Design review of the part built by this model. Coordinates are the model's own, in mm. Face numbers are marked on the shaded views. A direction names the side the tool comes from. Give positions to 0.01 mm unless a question says otherwise; leave off trailing zeros. Write each loop counter-clockwise with the first axis right and the second up, starting at its lowest first coordinate (ties: lowest second). Pieces come first, ordered by that corner, then holes. Notation, with made-up numbers: M -20,87 L -15,87 A25 ccw -15,120 Z; hole C 51.25,0 d1. An arc over 180 degrees is marked long. Answer in a Markdown table with one row per item.
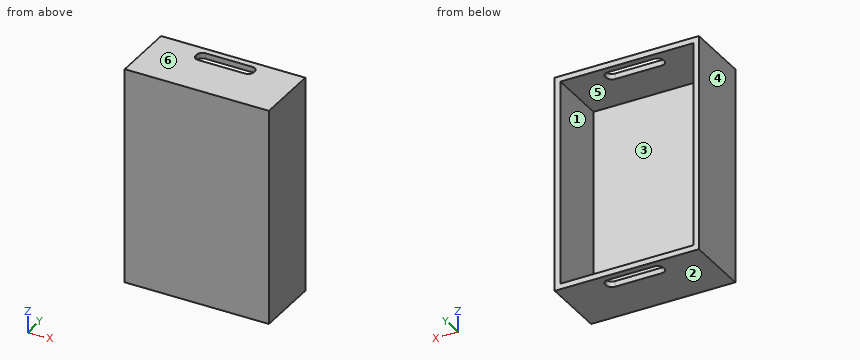
```python
from build123d import *

# Parameters (mm, degrees)
SKETCH1_W               = 385
SKETCH1_H               = 578
BOSS_EXTRUDE1_DEPTH     = 15
SKETCH2_W               = 15
SKETCH2_H               = 578
BOSS_EXTRUDE2_DEPTH     = 157.5
SKETCH3_W               = 355
SKETCH3_H               = 15
BOSS_EXTRUDE3_DEPTH     = 157.5
CUT_EXTRUDE1_DEPTH      = 634.16388084
CUT_EXTRUDE1_DEPTH_BACK = 634.16388084


with BuildPart() as part:
    # Sketch1 → Boss-Extrude1 (new body)
    with BuildSketch(Plane(origin=(0, 0, 0), x_dir=(1, 0, 0), z_dir=(0, 1, 0))):
        Rectangle(SKETCH1_W, SKETCH1_H)
    extrude(amount=BOSS_EXTRUDE1_DEPTH)

    # Sketch2 → Boss-Extrude2 (add)
    with BuildSketch(Plane(origin=(0, 15, 0), x_dir=(1, 0, 0), z_dir=(0, 1, 0))):
        with Locations((185, 0)):
            Rectangle(SKETCH2_W, SKETCH2_H)
    boss_extrude2 = extrude(amount=BOSS_EXTRUDE2_DEPTH)

    # Mirror1: Boss-Extrude2 across plane
    add(boss_extrude2.mirror(Plane(origin=(0, 0, 0), x_dir=(0, 0, 1), z_dir=(1, 0, 0))))

    # Sketch3 → Boss-Extrude3 (add)
    with BuildSketch(Plane(origin=(0, 15, 0), x_dir=(1, 0, 0), z_dir=(0, 1, 0))):
        with Locations((0, -281.5)):
            Rectangle(SKETCH3_W, SKETCH3_H)
    boss_extrude3 = extrude(amount=BOSS_EXTRUDE3_DEPTH)

    # Mirror2: Boss-Extrude3 across plane
    add(boss_extrude3.mirror(Plane.XY))

    # Sketch4 → Cut-Extrude1 (cut, two sides: drawn at the far end of the back side and taken through both)
    with BuildSketch(Plane.XY.offset(289).offset(-CUT_EXTRUDE1_DEPTH_BACK)):
        with BuildLine():
            Line((-64.034446869, 155), (60.965553131, 155))
            ThreePointArc((60.965553131, 155), (71.572154849, 150.606601718), (75.965553131, 140))
            Line((75.965553131, 140), (75.965553131, 135))
            ThreePointArc((75.965553131, 135), (71.572154849, 124.393398282), (60.965553131, 120))
            Line((60.965553131, 120), (-64.034446869, 120))
            ThreePointArc((-64.034446869, 120), (-74.641048586, 124.393398282), (-79.034446869, 135))
            Line((-79.034446869, 135), (-79.034446869, 140))
            ThreePointArc((-79.034446869, 140), (-74.641048586, 150.606601718), (-64.034446869, 155))
        make_face()
    extrude(amount=CUT_EXTRUDE1_DEPTH + CUT_EXTRUDE1_DEPTH_BACK, mode=Mode.SUBTRACT)


solid = part.part
```
1) To check wall thickness, follow probe 1 along X at (y, z) = (77.5, -117.5); probe 2 along Z at (x, y) = (-27, 16); probe 3 along Y at (x, z) = (116, 65.5). State the ranges of each line that lie inside material, in increasing order. Write a range as [from, to].
Geometry says:
| item | result |
|---|---|
| probe 1 | [-192.5, -177.5], [177.5, 192.5] |
| probe 2 | [-289, -274], [274, 289] |
| probe 3 | [0, 15] |
2) Add section C-C (y = 112.5). Write out the cut boundary in (x, z), and give its area (3 significant figures).
Geometry says:
| item | result |
|---|---|
| outline | M -192.5,-289 L 192.5,-289 L 192.5,289 L -192.5,289 Z; hole M -177.5,-274 L 177.5,-274 L 177.5,274 L -177.5,274 Z |
| area | 28,000 mm^2 |
3) Add section B-B (z = 32). Write out the cut boundary in (x, y).
Geometry says:
| item | result |
|---|---|
| outline | M -192.5,0 L 192.5,0 L 192.5,172.5 L 177.5,172.5 L 177.5,15 L -177.5,15 L -177.5,172.5 L -192.5,172.5 Z |
4) The part is to be moulded in two halves that separate along X. For the marked faces 3, 4, 5 and 6, say which applies: released by +X, released by -X, zero draft, split by the parting line, or undercut.
Geometry says:
| item | result |
|---|---|
| face 3 | undercut |
| face 4 | released by -X |
| face 5 | undercut |
| face 6 | zero draft |
5) Add section D-D (y = 146). Write out the cut boundary in (x, z).
Geometry says:
| item | result |
|---|---|
| outline | M -192.5,-289 L -77.78,-289 L -77.78,-274 L -177.5,-274 L -177.5,274 L -77.78,274 L -77.78,289 L -192.5,289 Z; M 74.71,-289 L 192.5,-289 L 192.5,289 L 74.71,289 L 74.71,274 L 177.5,274 L 177.5,-274 L 74.71,-274 Z |
6) Insertion check: P1, Ø1, axis at x = -100, z = -114.5, coming from the +Y side. The pin has a flat end and moves straight along its axis. Give the tip position at first contact, or say it passes through.
Geometry says:
| item | result |
|---|---|
| P1 | y = 15 |
7) For the marked faces 1 and 2, list the 3-axis set-ups (+Z, -Z, +X, -X, +Y, -Y) from which the entire face can be reached by the end or side of a thin tool; tool diameter is ignored.
Geometry says:
| item | result |
|---|---|
| face 1 | +Y |
| face 2 | -Z, +X, -X, +Y, -Y |
8) Add section A-A (x = 36). Write out the cut boundary in (y, z), and give its area (3 significant figures).
Geometry says:
| item | result |
|---|---|
| outline | M 0,-289 L 120,-289 L 120,-274 L 15,-274 L 15,274 L 120,274 L 120,289 L 0,289 Z; M 155,-289 L 172.5,-289 L 172.5,-274 L 155,-274 Z; M 155,274 L 172.5,274 L 172.5,289 L 155,289 Z |
| area | 12,300 mm^2 |
